from build123d import *

# Parameters (mm, degrees)
SKETCH1_W           = 30
SKETCH1_H           = 30
BOSS_EXTRUDE1_DEPTH = 15
FILLET1_R           = 4
CHAMFER2_SIZE       = 3
FILLET2_R           = 1
SKETCH3_R           = 10
BOSS_EXTRUDE2_DEPTH = 5
FILLET3_R           = 5
SKETCH4_W           = 5
SKETCH4_H           = 15
BOSS_EXTRUDE3_DEPTH = 20
CHAMFER3_SIZE       = 2
SKETCH5_R           = 5
CUT_EXTRUDE1_DEPTH  = 10
SKETCH6_R           = 0.75
BOSS_EXTRUDE5_DEPTH = 40
CIRPATTERN2_COUNT   = 8
SKETCH7_R           = 5
CUT_EXTRUDE2_DEPTH  = 10
CUT_EXTRUDE3_DEPTH  = 1
LPATTERN1_COUNT     = 2
LPATTERN1_PITCH     = 8
LPATTERN1_COL_COUNT = 2
LPATTERN1_COL_PITCH = 8


# Some blends are built 0.0001 mm under size
with BuildPart() as part:
    # Sketch1 → Boss-Extrude1 (new, symmetric)
    with BuildSketch(Plane.XY):
        Rectangle(SKETCH1_W, SKETCH1_H)
    extrude(amount=BOSS_EXTRUDE1_DEPTH, both=True)

    # Sketch2 → Revolve1 (revolve)
    with BuildSketch(Plane(origin=(0, 0, 0), x_dir=(0, 0, -1), z_dir=(1, 0, 0)), mode=Mode.PRIVATE) as revolve1_sk:
        Polygon((-55, 0), (-55, 15), (-52, 15), (-52, 9), (-15, 9), (-15, 0), align=None)
    revolve(revolve1_sk.sketch.rotate(Axis((0, 0, 15), (0, 0, 1)), 90), axis=Axis((0, 0, 15), (0, 0, 1)))

    # Fillet1
    fillet1_edges = [part.edges().sort_by_distance(p)[0] for p in [
        (15, -15, 0),
        (-15, -15, 0),
        (-15, 15, 0),
        (15, 15, 0),
    ]]
    fillet(fillet1_edges, radius=FILLET1_R)

    # Chamfer2
    # the kernel refuses this chamfer: 3 mm, written as the material it takes off along each edge
    with BuildSketch(Plane(origin=(15, 18.715048964, 15), x_dir=(-0.9996219169112969, 0, 0.02749587661058621), z_dir=(0, -1, 0))) as chamfer2_piece_1:
        Polygon((CHAMFER2_SIZE * 0.999621916911, CHAMFER2_SIZE * 0.0274958766106), (-CHAMFER2_SIZE * 0.0274958766106, CHAMFER2_SIZE * 0.999621916911), (0, 0), align=None)
    extrude(amount=37.430097928, mode=Mode.SUBTRACT)

    # Fillet2
    fillet2_edges = [part.edges().sort_by_distance(p)[0] for p in [
        (13.828427125, 13.828427125, -15),
        (15, 0, -15),
        (13.828427125, -13.828427125, -15),
        (0, -15, -15),
        (-13.828427125, -13.828427125, -15),
        (-15, 0, -15),
        (-13.828427125, 13.828427125, -15),
        (11.50401717, 14.968118785, 15),
        (11.50401717, -14.968118785, 15),
        (0, -15, 15),
        (-13.828427125, -13.828427125, 15),
        (-15, 0, 15),
        (-13.828427125, 13.828427125, 15),
        (0, 15, -15),
        (0, 15, 15),
    ]]
    fillet(fillet2_edges, radius=FILLET2_R)

    # Sketch3 → Boss-Extrude2 (add)
    with BuildSketch(Plane(origin=(0, 0, -15), x_dir=(-1, 0, 0), z_dir=(0, 0, -1))):
        with Locations(Location((0, 0, 0), (0, 0, 180))):
            Circle(SKETCH3_R)
    extrude(amount=BOSS_EXTRUDE2_DEPTH)

    # Fillet3
    fillet3_edges = [part.edges().sort_by_distance(p)[0] for p in [
        (-10, 0, -20),
    ]]
    fillet(fillet3_edges, radius=FILLET3_R - 0.0001)  # a hair under: the kernel refuses the full size

    # Sketch4 → Boss-Extrude3 (add)
    with BuildSketch(Plane(origin=(0, 0, -15), x_dir=(-1, 0, 0), z_dir=(0, 0, -1))):
        with Locations((-15, 0)):
            Rectangle(SKETCH4_W, SKETCH4_H)
    extrude(amount=-BOSS_EXTRUDE3_DEPTH)

    # Chamfer3
    chamfer3_edges = [part.edges().sort_by_distance(p)[0] for p in [
        (17.5, 7.5, -5),
        (17.5, 0, 5),
        (17.5, -7.5, -5),
    ]]
    chamfer(chamfer3_edges, length=CHAMFER3_SIZE)

    # Sketch5 → Cut-Extrude1 (cut)
    with BuildSketch(Plane.XY.offset(55)):
        Circle(SKETCH5_R)
    extrude(amount=-CUT_EXTRUDE1_DEPTH, mode=Mode.SUBTRACT)

    # Sketch6 → Boss-Extrude5 (add)
    with BuildSketch(Plane.XY.offset(55)):
        with Locations((0, 11)):
            Circle(SKETCH6_R)
    boss_extrude5 = extrude(amount=-BOSS_EXTRUDE5_DEPTH)

    # CirPattern2: Boss-Extrude5 ×8 about axis
    cirpattern2_axis = Axis((0, 0, 0), (0, 0, 1))
    for i in range(1, CIRPATTERN2_COUNT):
        add(boss_extrude5.rotate(cirpattern2_axis, i * 360 / CIRPATTERN2_COUNT))

    # Sketch7 → Cut-Extrude2 (cut)
    with BuildSketch(Plane.ZY.offset(15)):
        with Locations(Location((0, 0, 0), (0, 0, 270))):
            Circle(SKETCH7_R)
    extrude(amount=-CUT_EXTRUDE2_DEPTH, mode=Mode.SUBTRACT)

    # Sketch8 → Cut-Extrude3 (cut)
    with BuildSketch(Plane(origin=(0, 15, 0), x_dir=(1, 0, 0), z_dir=(0, 1, 0))):
        with BuildLine():
            Line((-1, -10), (-1, 10))
            ThreePointArc((-1, 10), (0, 11), (1, 10))
            Line((1, 10), (1, -10))
            ThreePointArc((1, -10), (0, -11), (-1, -10))
        make_face()
    cut_extrude3 = extrude(amount=-CUT_EXTRUDE3_DEPTH, mode=Mode.SUBTRACT)

    # LPattern1: Cut-Extrude3 ×2
    with Locations(*[(-i * LPATTERN1_PITCH, 0, 0) for i in range(1, LPATTERN1_COUNT)]):
        add(cut_extrude3, mode=Mode.SUBTRACT)

    # LPattern1 col: Cut-Extrude3 ×2
    with Locations(*[(i * LPATTERN1_COL_PITCH, 0, 0) for i in range(1, LPATTERN1_COL_COUNT)]):
        add(cut_extrude3, mode=Mode.SUBTRACT)


solid = part.part
Read the model definition and answer for the solid it produces. Units are mm, in the model's axes. A direction names the side the tool comes from. Round coordinates to 2 decimals unless told otherwise and drop trailing zeros.
1) The part is cut by section A-A on z = 33. Give the number of separate pieces and of enclosed holes in the cut face, plus the area to 3 significant figures.
2) Flat-ended cylindrical pins translate along their axes: pin 1 (1.1 mm diameter, centred on y = 14.5, z = -3.5, fed in from +X); pin 2 (0.5 mm diameter, centred on y = 14.5, z = 2, fed in from -X); pin 3 (8 mm diameter, centred on y = 2.5, z = 10, fed in from +X). Find the tip coordinate at first contact, or state that the pin passes through.
3) Straight lines are drawn through the part: L1, parallel to Y at x = 0, z = 50; L2, parallel to Z at x = -9.5, y = 10.5; L3, parallel to Z at x = 13, y = -6. For each, find the intervals that lie inside material, in ascending order.
4) The mould has two halves that part along Z. Classify faces 5 (the face through (16.5, -0.1, 4)), 6 (the face through (6.633, -6.083, 33.241)), 7 (the face through (15, 0, 8)), 8 (the face through (0, 0, -20)): released by +Z, released by -Z, zero draft, split by the parting line, or undercut.
5) For faces 1 (the face through (-5, 0, 0)), 2 (the face through (-1.08, -4.88, 50.07)), 3 (the face through (8, 14, 0)), 4 (the face through (-6.5, 6.5, 52)), determine the directions among +Z, -Z, +X, -X, +Y, -Y from which every point of the face is accessible in a straight line to the end or side of a thin tool.
Resolved:
1. separate pieces: 9
1. enclosed holes: 0
1. area: 269 mm2
2. pin 1: stops at x = 13.7
2. pin 2: stops at x = -13.33
2. pin 3: stops at x = 15
3. L1: y = -11.75 to -10.25, -9 to -5, 5 to 9, 10.25 to 11.75
3. L2: z = -15 to 15, 52 to 55
3. L3: z = -15 to 14, 52 to 55
4. face 5: released by +Z
4. face 6: undercut
4. face 7: zero draft
4. face 8: released by -Z
5. face 1: -X
5. face 2: +Z
5. face 3: +Y
5. face 4: none
